```python
from build123d import *

# Parameters (mm, degrees)
SKETCH1_W           = 20
SKETCH1_H           = 40
SKETCH1_W_2         = 50
SKETCH1_H_2         = 65
SKETCH1_R           = 2.25
BOSS_EXTRUDE1_DEPTH = 10.5
SKETCH3_R           = 6.5
SKETCH3_R_2         = 8
BOSS_EXTRUDE2_DEPTH = 8
SKETCH4_R           = 3.75
CUT_EXTRUDE1_DEPTH  = 6
SKETCH5_R           = 18
BOSS_EXTRUDE3_DEPTH = 12.3
SKETCH7_W           = 167.229187532
SKETCH7_H           = 99.836007656
SKETCH7_R           = 15
CUT_EXTRUDE2_DEPTH  = 7
SKETCH8_R           = 21
BOSS_EXTRUDE4_DEPTH = 78
CHAMFER1_SIZE       = 1
SKETCH9_R           = 2
BOSS_EXTRUDE5_DEPTH = 3


with BuildPart() as part:
    # Sketch1 → Boss-Extrude1 (new body)
    with BuildSketch(Plane.XY):
        Polygon((-25, -20), (-45, -20), (-25, -32.5), align=None)
        with Locations((-35, 0)):
            Rectangle(SKETCH1_W, SKETCH1_H)
        Polygon((-25, 20), (-25, 32.5), (-45, 20), align=None)
        Rectangle(SKETCH1_W_2, SKETCH1_H_2)
        with Locations((-3, 26)):
            Circle(SKETCH1_R, mode=Mode.SUBTRACT)
        with Locations((-3, -26)):
            Circle(SKETCH1_R, mode=Mode.SUBTRACT)
    boss_extrude1 = extrude(amount=BOSS_EXTRUDE1_DEPTH)

    # Mirror1: Boss-Extrude1 across plane
    add(boss_extrude1.mirror(Plane(origin=(25, 0, 10.5), x_dir=(0, 0, 1), z_dir=(1, 0, 0))))

    # Sketch3 → Boss-Extrude2 (add)
    with BuildSketch(Plane.XY.offset(10.5)):
        with Locations((25, 0)):
            Circle(SKETCH3_R)
        with Locations((-30, -9.5)):
            Circle(SKETCH3_R_2)
        with Locations((80, -9.5)):
            Circle(SKETCH3_R_2)
    extrude(amount=BOSS_EXTRUDE2_DEPTH)

    # Sketch4 → Cut-Extrude1 (cut)
    with BuildSketch(Plane.XY.offset(10.5)):
        with Locations((-3, -26)):
            Circle(SKETCH4_R)
        with Locations((-3, 26)):
            Circle(SKETCH4_R)
        with Locations((53, 26)):
            Circle(SKETCH4_R)
        with Locations((53, -26)):
            Circle(SKETCH4_R)
    extrude(amount=-CUT_EXTRUDE1_DEPTH, mode=Mode.SUBTRACT)

    # Sketch5 → Boss-Extrude3 (add)
    with BuildSketch(Plane.XY.offset(18.5)):
        with Locations((25, 0)):
            Circle(SKETCH5_R)
        with Locations((-30, -9.5)):
            Circle(SKETCH5_R)
    extrude(amount=BOSS_EXTRUDE3_DEPTH)

    # Sketch7 → Cut-Extrude2 (cut)
    with BuildSketch(Plane.XY.offset(28.3)):
        with Locations((-30, -9.5)):
            Rectangle(SKETCH7_W, SKETCH7_H)
        with Locations((-30, -9.5)):
            Circle(SKETCH7_R, mode=Mode.SUBTRACT)
        with Locations((25, 0)):
            Circle(SKETCH7_R, mode=Mode.SUBTRACT)
    extrude(amount=-CUT_EXTRUDE2_DEPTH, mode=Mode.SUBTRACT)

    # Mirror2: part across plane


with BuildPart() as part_1:
    add(part.part)
    add(part.part.mirror(Plane(origin=(25, 0, 0), x_dir=(0, 0, 1), z_dir=(1, 0, 0))))

    # Sketch8 → Boss-Extrude4 (add)
    with BuildSketch(Plane(origin=(0, 0, 0), x_dir=(-1, 0, 0), z_dir=(0, 0, -1))):
        with Locations((-25, 0)):
            Circle(SKETCH8_R)
    extrude(amount=BOSS_EXTRUDE4_DEPTH)

    # Chamfer1
    chamfer1_edges = [part_1.edges().sort_by_distance(p)[0] for p in [
        (46, 0, -78),
    ]]
    chamfer(chamfer1_edges, length=CHAMFER1_SIZE)

    # Sketch9 → Boss-Extrude5 (add, symmetric)
    with BuildSketch(Plane(origin=(0, 0, 0), x_dir=(-1, 0, 0), z_dir=(0, 0, -1))):
        with Locations((-80, -9.5)):
            Circle(SKETCH9_R)
        with Locations((30, -9.5)):
            Circle(SKETCH9_R)
    extrude(amount=BOSS_EXTRUDE5_DEPTH, both=True)


solid = part_1.part
```
CAD build for the part. Positions are in the model's coordinates, mm. A direction names the side the tool comes from. Round coordinates to 2 decimals unless told otherwise and drop trailing zeros. Write each loop counter-clockwise with the first axis right and the second up, starting at its lowest first coordinate (ties: lowest second). Pieces come first, ordered by that corner, then holes.
Item 1: Band-saw the part on B-B on z = -6.5. Write the cut outline in (x, y).
Filled in:
outline: circle Ø42 at (25, 0)
Item 2: Band-saw the part on C-C on x = 80. Write the cut outline in (y, z) (3 decimals).
Filled in:
outline: (-29.375, 0) - (-11.5, 0) - (-11.5, -3) - (-7.5, -3) - (-7.5, 0) - (29.375, 0) - (29.375, 10.5) - (-1.5, 10.5) - (-1.5, 18.5) - (8.5, 18.5) - (8.5, 21.3) - (5.5, 21.3) - (5.5, 28.3) - (8.5, 28.3) - (8.5, 30.8) - (-27.5, 30.8) - (-27.5, 28.3) - (-24.5, 28.3) - (-24.5, 21.3) - (-27.5, 21.3) - (-27.5, 18.5) - (-17.5, 18.5) - (-17.5, 10.5) - (-29.375, 10.5) - close
Item 3: Tool access for faces 4 (the cylindrical face through (54.73, -29.327, 7.542)), 5 (the flat face through (80, -9, -3)), 6 (the cylindrical face through (73.651, -14.368, 14.444)): list every direction of +Z, -Z, +X, -X, +Y, -Y with a clear straight run to the whole face (end or side of a thin tool).
Filled in:
face 4: +Z
face 5: -Z, +X, +Y, -Y
face 6: none
Item 4: Drop flat-ended pins along their axis: pin 1 Ø8 at (y, z) = (2, -16) entering from -X; pin 2 Ø7 at (x, y) = (53, 26) entering from -Z; pin 3 Ø5 at (x, y) = (53, -26) entering from +Z. Give the stop position or say it passes through.
Filled in:
pin 1: stops at x = 4
pin 2: stops at z = 0
pin 3: stops at z = 4.5
Item 5: Band-saw the part on A-A on x = 53. Write the cut outline in (y, z).
Filled in:
outline: (-32.5, 0) - (-28.25, 0) - (-28.25, 4.5) - (-29.75, 4.5) - (-29.75, 10.5) - (-32.5, 10.5) - close; (-23.75, 0) - (23.75, 0) - (23.75, 4.5) - (22.25, 4.5) - (22.25, 10.5) - (-22.25, 10.5) - (-22.25, 4.5) - (-23.75, 4.5) - close; (28.25, 0) - (32.5, 0) - (32.5, 10.5) - (29.75, 10.5) - (29.75, 4.5) - (28.25, 4.5) - close
Item 6: Mould opens along X. For faces 1 (the flat face through (-34.86, 26.338, 5.176)), 2 (the flat face through (25, 0, -78)), 3 (the flat face through (72, -13, 18.5)) say: released by +X, released by -X, zero draft, split by the parting line, or undercut.
Filled in:
face 1: released by -X
face 2: zero draft
face 3: undercut
Item 7: Drill centre lines: L1, parallel to Y at x = -3, z = 7.6; L2, parallel to Y at x = -3, z = 2; L3, parallel to Z at x = -32.5, y = -26. Where is each one in solid material? Low to high.
Filled in:
L1: y = -32.5 to -29.75, -22.25 to 22.25, 29.75 to 32.5
L2: y = -32.5 to -28.25, -23.75 to 23.75, 28.25 to 32.5
L3: z = 0 to 10.5, 18.5 to 21.3, 28.3 to 30.8
